Could you check a few things on this drawing? It's one solid part, dimensions in mm from its lowest x, y, z. Coordinates: 2 decimals unless noted, no trailing zeros. Order: outer loops, then holes, each group sorted by start corner. A loop starts at its lowest first (then second) coordinate and runs counter-clockwise, first axis right, second up. Notation, with made-up numbers: (-8.5, -21) - (-3.5, -21) arc R21 ccw to (-3.5, 16) - close; hole circle Ø3 at (-35.75, 11.5). An arc over 180 degrees is marked (long way). Answer in a Markdown table with one row per item. Add a question column.
Item 1: I want a section at D-D (z = 12.5). Please give me the cut outline in (x, y).
Item 2: I want a section at B-B (z = 36.5). Please give me the cut outline in (x, y), plus the area to 3 significant figures.
Item 3: I want a section at A-A (x = 5.5). Please give me the cut outline in (y, z).
Item 4: I want a section at C-C (y = 1.4). Count the separate pieces of the cut face and the enclosed holes in it, plus the area to 3 significant figures.
Item 5: If I drill on line 1 along X through (y, z) = (0.7, 5.5); line 2 along X through (y, z) = (1.55, 21); line 3 along Z through (x, y) = (36.5, 0.6), over which ranges is the centre line in solid material (lowest first)? Write a range as from..to.
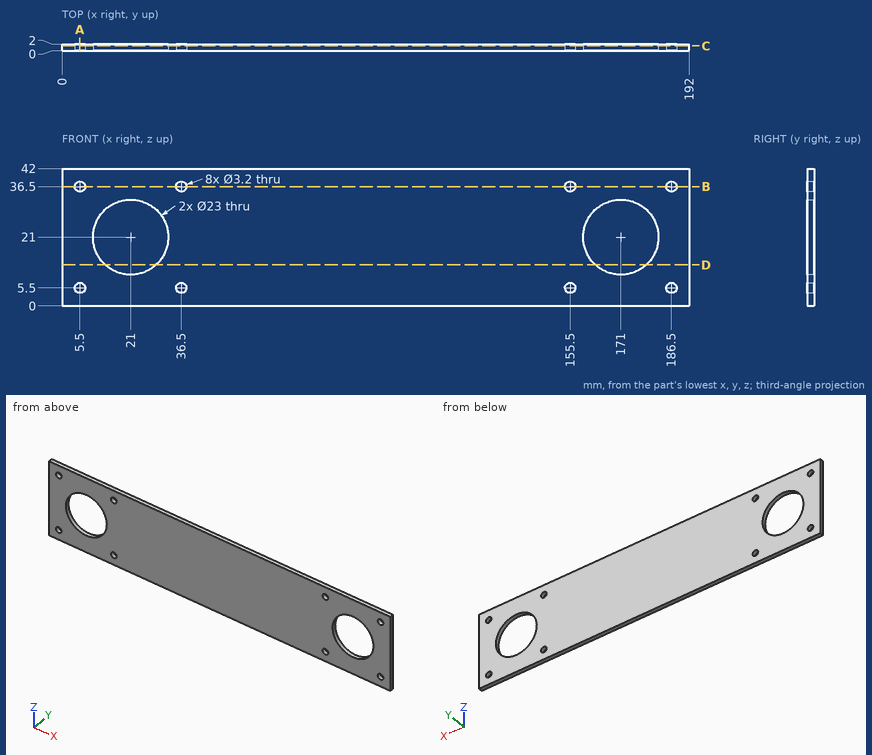
Values follow:
| question | item | result |
|---|---|---|
| 1 | outline | (0, 0) - (13.25, 0) - (13.25, 2) - (0, 2) - close; (28.75, 0) - (163.25, 0) - (163.25, 2) - (28.75, 2) - close; (178.75, 0) - (192, 0) - (192, 2) - (178.75, 2) - close |
| 2 | outline | (0, 0) - (3.9, 0) - (3.9, 2) - (0, 2) - close; (7.1, 0) - (34.9, 0) - (34.9, 2) - (7.1, 2) - close; (38.1, 0) - (153.9, 0) - (153.9, 2) - (38.1, 2) - close; (157.1, 0) - (184.9, 0) - (184.9, 2) - (157.1, 2) - close; (188.1, 0) - (192, 0) - (192, 2) - (188.1, 2) - close |
| 2 | area | 358 mm^2 |
| 3 | outline | (0, 0) - (2, 0) - (2, 3.9) - (0, 3.9) - close; (0, 7.1) - (2, 7.1) - (2, 34.9) - (0, 34.9) - close; (0, 38.1) - (2, 38.1) - (2, 42) - (0, 42) - close |
| 4 | separate pieces | 1 |
| 4 | enclosed holes | 10 |
| 4 | area | 7,170 mm^2 |
| 5 | line 1 | x = 0..3.9, 7.1..34.9, 38.1..153.9, 157.1..184.9, 188.1..192 |
| 5 | line 2 | x = 0..9.5, 32.5..159.5, 182.5..192 |
| 5 | line 3 | z = 0..3.9, 7.1..34.9, 38.1..42 |
